Input: dimensioned drawing with shaded views. Units: mm. Origin: part minimum x, y, z. Round coordinates to 2 decimals unless told otherwise and drop trailing zeros. Loops run counter-clockwise (first coordinate to the right, second up) from the corner with the lowest first, then second, coordinate; pieces in that order, holes last. Notation, with made-up numbers: (-33.5, 19) -> (-7.5, 19) arc R8 ccw to (-7.5, 25) -> close; hole circle Ø9 at (36.25, 43). An arc over 180 degrees is marked (long way). Answer as a JSON object with one key per item and string values.
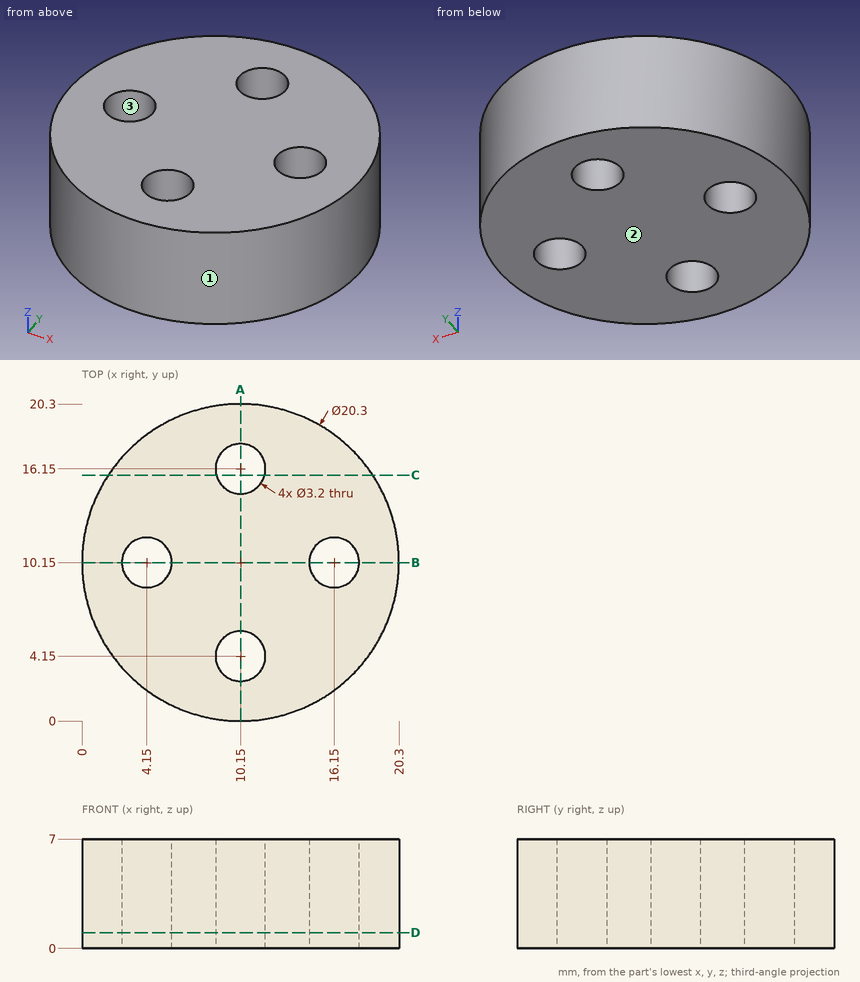
1) Section D-D, the plane z = 1. Output: boundary loops of the cut face in (x, y).
Output:
{"outline": "circle Ø20.3 at (10.15, 10.15); hole circle Ø3.2 at (4.15, 10.15); hole circle Ø3.2 at (10.15, 4.15); hole circle Ø3.2 at (10.15, 16.15); hole circle Ø3.2 at (16.15, 10.15)"}
2) Contact query for flat-ended pins moving along their axis: P1, Ø1, axis at x = 18, z = 4, coming from the -Y side; P2, Ø1.5, axis at y = 12, z = 4, coming from the -X side. Output: stop coordinate, or through.
Output:
{"P1": "stops at y = 3.15", "P2": "stops at x = 0.06"}
3) Section A-A, the plane x = 10.15. Output: boundary loops of the cut face in (y, z), plus the area to 3 significant figures.
Output:
{"outline": "(0, 0) -> (2.55, 0) -> (2.55, 7) -> (0, 7) -> close; (5.75, 0) -> (14.55, 0) -> (14.55, 7) -> (5.75, 7) -> close; (17.75, 0) -> (20.3, 0) -> (20.3, 7) -> (17.75, 7) -> close", "area": "97.3 mm^2"}
4) Ray query, probe 1 along Y at (x, z) = (10.15, 3); probe 2 along X at (y, z) = (11.25, 5). Return the intervals inside material, ascending.
Output:
{"probe 1": "y = 0 to 2.55, 5.75 to 14.55, 17.75 to 20.3", "probe 2": "x = 0.06 to 2.99, 5.31 to 14.99, 17.31 to 20.24"}
5) Draft query along X for the marked faces 1, 2 and 3. Return one class per face: +X half, -X half, draft (parallel to the pull), parting line (faces both ways), or undercut.
Output:
{"face 1": "parting line", "face 2": "draft", "face 3": "undercut"}
6) Section C-C, the plane y = 15.75. Output: boundary loops of the cut face in (x, z).
Output:
{"outline": "(1.68, 0) -> (8.6, 0) -> (8.6, 7) -> (1.68, 7) -> close; (11.7, 0) -> (18.62, 0) -> (18.62, 7) -> (11.7, 7) -> close"}
